Part model, mm, in its own coordinate system. A direction names the side the tool comes from. Round coordinates to 2 decimals unless told otherwise and drop trailing zeros. Loops run counter-clockwise (first coordinate to the right, second up) from the corner with the lowest first, then second, coordinate; pieces in that order, holes last. Notation, with made-up numbers: (29.25, 63) -> (46.25, 63) arc R27 ccw to (46.25, 83) -> close; hole circle Ø7 at (10, 63.25). An arc over 180 degrees is marked (long way). Use a Markdown table: item, result. Add a question column.
Item 1: Cut at B-B, the plane x = 1. List the corners of the cut face in (y, z).
Item 2: Probe line 1 (Y direction, x = -5.5, z = 10.5); line 2 (X direction, y = 3.75, z = 10); line 3 (Z direction, x = 13, y = -0.75). List the from-to ranges inside material, lowest first. Write a range as [from, to].
Item 3: Which spindle directions (+Z, -Z, +X, -X, +Y, -Y) get a long thin tool onto all of the face, cutting with end or side? Do faces 5 (the face through (0, -0.074, 1)), 6 (the face through (10.922, 0, 8)), 7 (the face through (-15.975, 2.901, 18.479)), 8 (the face through (0, -1, 1.4)). Say none if no direction does.
Item 4: Two-plate mould, pull along Y, no slides. Class faces 1 (the face through (-10.6, 0.2, 17)), 2 (the face through (-9.678, 0, 11)), 3 (the face through (17, -1, 20)), 4 (the face through (19.42, -0.06, 19.03)): pulls with the +Y half, pulls with the -Y half, needs draft (parallel to the pull), parting line crosses it, or undercut.
Item 5: Cut at A-A, the plane z = 4.5. List the corners of the cut face in (x, y).
Item 6: Cut at C-C, the plane y = -0.75. List the corners of the cut face in (x, z), plus the area to 3 significant figures.
Item 7: Cut at D-D, the plane x = -9. List the corners of the cut face in (y, z).
Item 8: Flat gauge pins, fed straight in: pin 1 (10 mm diameter, centred on x = -6, z = 8.5, fed in from +Y); pin 2 (2.5 mm diameter, centred on y = 0.5, z = 18, fed in from -X); pin 3 (2.5 mm diameter, centred on x = -14, y = 0.5, fed in from -Z); pin 4 (1 mm diameter, centred on x = 13, z = 7.5, fed in from -Y). Where does each tip first touch, or does it go through?
```python
from build123d import *

# Parameters (mm, degrees)
SKETCH1_W           = 21
SKETCH1_H           = 9.65
BOSS_EXTRUDE1_DEPTH = 21
SKETCH3_W           = 20.2
SKETCH3_H           = 7.65
CUT_EXTRUDE1_DEPTH  = 19.6
CUT_EXTRUDE2_DEPTH  = 19.6
BOSS_EXTRUDE2_DEPTH = 4
CUT_EXTRUDE3_DEPTH  = 3
SKETCH22_R          = 1.65
CUT_EXTRUDE4_DEPTH  = 3
BOSS_EXTRUDE3_DEPTH = 4
CUT_EXTRUDE5_DEPTH  = 3
SKETCH25_R          = 1.65
CUT_EXTRUDE6_DEPTH  = 3


with BuildPart() as part:
    # Sketch1 → Boss-Extrude1 (new body)
    with BuildSketch(Plane.XY):
        with Locations((0.42161215, 0.10146028)):
            Rectangle(SKETCH1_W, SKETCH1_H)
    extrude(amount=BOSS_EXTRUDE1_DEPTH)

    # Sketch3 → Cut-Extrude1 (cut)
    with BuildSketch(Plane.XY.offset(21)):
        with Locations((0.42161215, 0.10146028)):
            Rectangle(SKETCH3_W, SKETCH3_H)
    extrude(amount=-CUT_EXTRUDE1_DEPTH, mode=Mode.SUBTRACT)

    # Sketch5 → Cut-Extrude2 (cut)
    with BuildSketch(Plane.XY.offset(1.4)):
        with BuildLine():
            Line((-0.82838785, 3.92646028), (1.67161215, 3.92646028))
            ThreePointArc((1.67161215, 3.92646028), (3.67161215, 1.92646028), (1.67161215, -0.07353972))
            Line((1.67161215, -0.07353972), (-0.82838785, -0.07353972))
            ThreePointArc((-0.82838785, -0.07353972), (-2.82838785, 1.92646028), (-0.82838785, 3.92646028))
        make_face()
    extrude(amount=-CUT_EXTRUDE2_DEPTH, mode=Mode.SUBTRACT)

    # Sketch20 → Boss-Extrude2 (add)
    with BuildSketch(Plane.XY.offset(21)):
        with BuildLine():
            Line((-10.07838785, -4.72353972), (-10.07838785, 4.92646028))
            ThreePointArc((-10.07838785, 4.92646028), (-18.57838785, 0.10146028), (-10.07838785, -4.72353972))
        make_face()
    extrude(amount=-BOSS_EXTRUDE2_DEPTH)

    # Sketch21 → Cut-Extrude3 (cut)
    with BuildSketch(Plane(origin=(0, 0, 17), x_dir=(-1, 0, 0), z_dir=(0, 0, -1))):
        Polygon((14.32838785, 3.85146028), (11.080792586, 1.97646028), (11.080792586, -1.77353972), (14.32838785, -3.64853972), (17.575983115, -1.77353972), (17.575983115, 1.97646028), align=None)
    extrude(amount=-CUT_EXTRUDE3_DEPTH, mode=Mode.SUBTRACT)

    # Sketch22 → Cut-Extrude4 (cut)
    with BuildSketch(Plane(origin=(0, 0, 20), x_dir=(-1, 0, 0), z_dir=(0, 0, -1))):
        with Locations((14.32838785, 0.10146028)):
            Circle(SKETCH22_R)
    extrude(amount=-CUT_EXTRUDE4_DEPTH, mode=Mode.SUBTRACT)

    # Sketch23 → Boss-Extrude3 (add)
    with BuildSketch(Plane.XY.offset(21)):
        with BuildLine():
            Line((10.92161215, 4.92646028), (10.92161215, -4.72353972))
            ThreePointArc((10.92161215, -4.72353972), (19.42161215, 0.10146028), (10.92161215, 4.92646028))
        make_face()
    extrude(amount=-BOSS_EXTRUDE3_DEPTH)

    # Sketch24 → Cut-Extrude5 (cut)
    with BuildSketch(Plane(origin=(0, 0, 17), x_dir=(-1, 0, 0), z_dir=(0, 0, -1))):
        Polygon((-15.17161215, 3.85146028), (-18.419207414, 1.97646028), (-18.419207414, -1.77353972), (-15.17161215, -3.64853972), (-11.924016885, -1.77353972), (-11.924016885, 1.97646028), align=None)
    extrude(amount=-CUT_EXTRUDE5_DEPTH, mode=Mode.SUBTRACT)

    # Sketch25 → Cut-Extrude6 (cut)
    with BuildSketch(Plane(origin=(0, 0, 20), x_dir=(-1, 0, 0), z_dir=(0, 0, -1))):
        with Locations((-15.17161215, 0.10146028)):
            Circle(SKETCH25_R)
    extrude(amount=-CUT_EXTRUDE6_DEPTH, mode=Mode.SUBTRACT)


solid = part.part
```
A:
| question | item | result |
|---|---|---|
| 1 | outline | (-4.72, 0) -> (-0.07, 0) -> (-0.07, 1.4) -> (-3.72, 1.4) -> (-3.72, 21) -> (-4.72, 21) -> close; (3.93, 0) -> (4.93, 0) -> (4.93, 21) -> (3.93, 21) -> close |
| 2 | line 1 | y = [-4.72, -3.72], [3.93, 4.93] |
| 2 | line 2 | x = [-10.08, -9.68], [10.52, 10.92] |
| 2 | line 3 | z = [20, 21] |
| 3 | face 5 | +Z, -Z |
| 3 | face 6 | -Z, +X, +Y, -Y |
| 3 | face 7 | -Z |
| 3 | face 8 | +Z |
| 4 | face 1 | needs draft |
| 4 | face 2 | undercut |
| 4 | face 3 | undercut |
| 4 | face 4 | parting line crosses it |
| 5 | outline | (-10.08, -4.72) -> (10.92, -4.72) -> (10.92, 4.93) -> (-10.08, 4.93) -> close; hole (-9.68, -3.72) -> (10.52, -3.72) -> (10.52, 3.93) -> (-9.68, 3.93) -> close |
| 6 | outline | (-18.51, 17) -> (-17.58, 17) -> (-17.58, 20) -> (-15.74, 20) -> (-15.74, 21) -> (-18.51, 21) -> close; (-12.92, 20) -> (-11.08, 20) -> (-11.08, 17) -> (-10.08, 17) -> (-10.08, 0) -> (10.92, 0) -> (10.92, 17) -> (11.92, 17) -> (11.92, 20) -> (13.76, 20) -> (13.76, 21) -> (10.52, 21) -> (10.52, 1.4) -> (-9.68, 1.4) -> (-9.68, 21) -> (-12.92, 21) -> close; (16.58, 20) -> (18.42, 20) -> (18.42, 17) -> (19.36, 17) -> (19.36, 21) -> (16.58, 21) -> close |
| 6 | area | 67.9 mm^2 |
| 7 | outline | (-4.72, 0) -> (4.93, 0) -> (4.93, 21) -> (3.93, 21) -> (3.93, 1.4) -> (-3.72, 1.4) -> (-3.72, 21) -> (-4.72, 21) -> close |
| 8 | pin 1 | stops at y = 4.93 |
| 8 | pin 2 | stops at x = -18.58 |
| 8 | pin 3 | stops at z = 20 |
| 8 | pin 4 | passes through |
